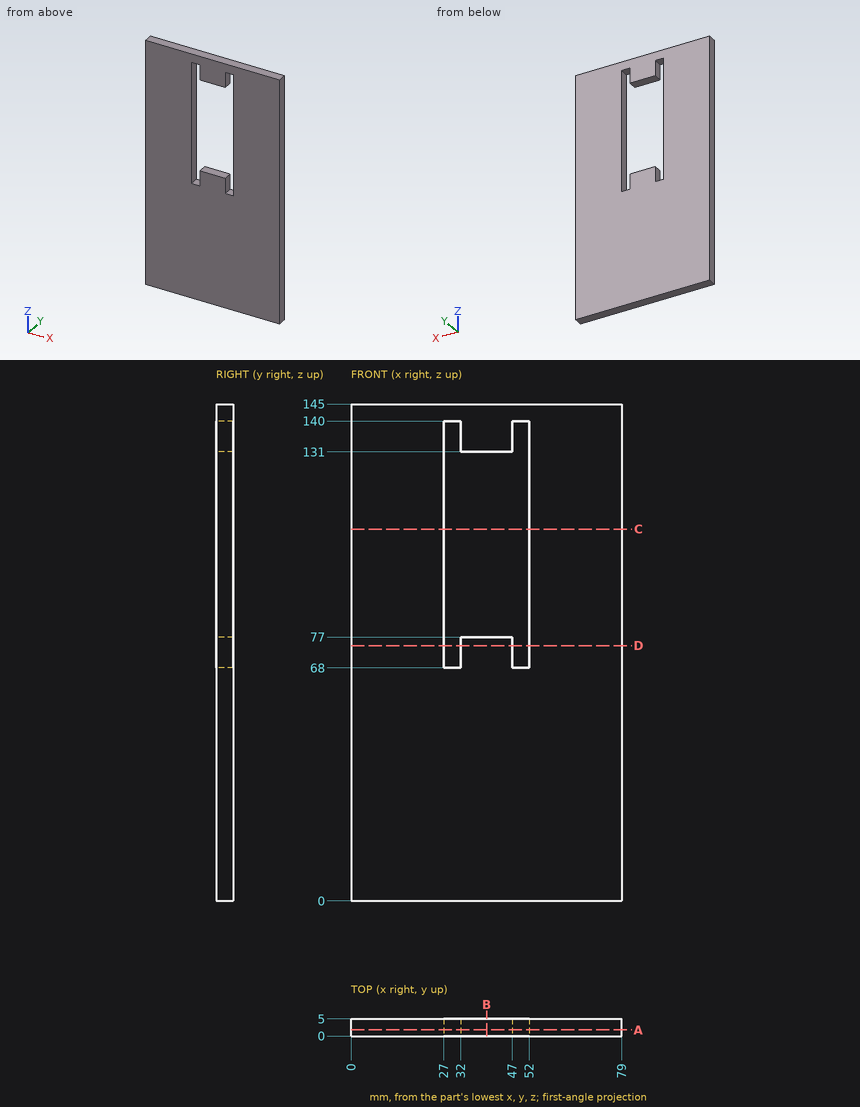
For this review, use the dimensioned drawing (mm, ordinates from the lowest corner) and the shaded views. Coordinates: 2 decimals unless noted, no trailing zeros. Order: outer loops, then holes, each group sorted by start corner. A loop starts at its lowest first (then second) coordinate and runs counter-clockwise, first axis right, second up. Notation, with made-up numbers: (48, 20.25) - (89, 20.25) arc R24 cw to (89, 40.25) - close; hole circle Ø5 at (29, 23.25). An arc over 180 degrees is marked (long way). Answer as a JSON object with one key per item and string values. Group by question number.
1. We need section D-D on z = 74.5. State the section outline as (x, y) points.
2. We need section C-C on z = 108.5. State the section outline as (x, y) points, then the cut area to 3 significant figures.
3. For probe 1 along X at (y, z) = (4.4, 132.5); probe 2 along X at (y, z) = (1.3, 124); probe 3 along Z at (x, y) = (33.5, 2.7), list the stretches that pass through material, from the lowest coordinate up.
4. We need section A-A on y = 1.8. State the section outline as (x, z) points, then the cut area to 4 significant figures.
5. Clearance check with a flat-ended pin moving along its axis: P1, Ø1.5, axis at y = 1.5, z = 73, coming from the -X side. State where the tip first meets the part, or that it passes through.
6. We need section B-B on x = 39.5. State the section outline as (y, z) points, then the cut area to 3 significant figures.
Final values:
{
 "1": {"outline": "(0, 0) - (27, 0) - (27, 5) - (0, 5) - close; (32, 0) - (47, 0) - (47, 5) - (32, 5) - close; (52, 0) - (79, 0) - (79, 5) - (52, 5) - close"},
 "2": {"outline": "(0, 0) - (27, 0) - (27, 5) - (0, 5) - close; (52, 0) - (79, 0) - (79, 5) - (52, 5) - close", "area": "270 mm²"},
 "3": {"probe 1": "0 to 27, 32 to 47, 52 to 79", "probe 2": "0 to 27, 52 to 79", "probe 3": "0 to 77, 131 to 145"},
 "4": {"outline": "(0, 0) - (79, 0) - (79, 145) - (0, 145) - close; hole (27, 68) - (32, 68) - (32, 77) - (47, 77) - (47, 68) - (52, 68) - (52, 140) - (47, 140) - (47, 131) - (32, 131) - (32, 140) - (27, 140) - close", "area": "9,925 mm²"},
 "5": {"P1": "x = 0"},
 "6": {"outline": "(0, 0) - (5, 0) - (5, 77) - (0, 77) - close; (0, 131) - (5, 131) - (5, 145) - (0, 145) - close", "area": "455 mm²"}
}
